Check sheet for the modelled part. Datum: model origin and axes. Units: mm. Round coordinates to 2 decimals unless told otherwise and drop trailing zeros. Write each loop counter-clockwise with the first axis right and the second up, starting at its lowest first coordinate (ties: lowest second). Pieces come first, ordered by that corner, then holes. Notation, with made-up numbers: M 68,43.25 L 75,43.25 A31 cw 75,76.25 Z; hole C 2,6.25 d3. An arc over 180 degrees is marked long. Answer in a Markdown table with one row per item.
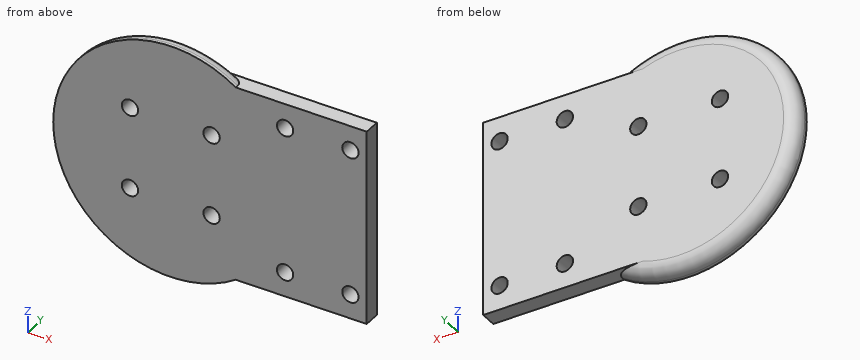
```python
from build123d import *

# Parameters (mm, degrees)
EXTRUDE_1_DEPTH     = 5
FILLET_1_R          = 4
SKETCH_2_R          = 2.5
CUT_EXTRUDE_1_DEPTH = 71.149839773


with BuildPart() as part:
    # 草图1 → 凸台-拉伸1 (new body)
    with BuildSketch(Plane(origin=(0, 0, 0), x_dir=(1, 0, 0), z_dir=(0, 1, 0))):
        with BuildLine():
            Line((19.899748742, -30), (60, -30))
            Line((60, -30), (60, 30))
            Line((60, 30), (19.899748742, 30))
            ThreePointArc((19.899748742, 30), (-36, 0), (19.899748742, -30))
        make_face()
    extrude(amount=EXTRUDE_1_DEPTH)

    # 圆角1
    fillet_1_edges = [part.edges().sort_by_distance(p)[0] for p in [
        (-36, 5, 0),
    ]]
    fillet(fillet_1_edges, radius=FILLET_1_R)

    # 草图2 → 切除-拉伸1 (cut, through all)
    with BuildSketch(Plane(origin=(0, 5, 0), x_dir=(1, 0, 0), z_dir=(0, 1, 0))):
        with Locations(Location((-12.5, 12.5, 0), (0, 0, 270))):
            Circle(SKETCH_2_R)
        with Locations(Location((12.5, 12.5, 0), (0, 0, 270))):
            Circle(SKETCH_2_R)
        with Locations(Location((12.5, -12.5, 0), (0, 0, 270))):
            Circle(SKETCH_2_R)
        with Locations(Location((-12.5, -12.5, 0), (0, 0, 270))):
            Circle(SKETCH_2_R)
        with Locations(Location((35, 22.5, 0), (0, 0, 270))):
            Circle(SKETCH_2_R)
        with Locations(Location((55, 22.5, 0), (0, 0, 270))):
            Circle(SKETCH_2_R)
        with Locations(Location((55, -22.5, 0), (0, 0, 270))):
            Circle(SKETCH_2_R)
        with Locations(Location((35, -22.5, 0), (0, 0, 270))):
            Circle(SKETCH_2_R)
    extrude(amount=-CUT_EXTRUDE_1_DEPTH, mode=Mode.SUBTRACT)


solid = part.part
```
1. Section check D-D, the plane x = 39.5. Record the cut outline in (y, z).
Found:
| item | result |
|---|---|
| outline | M 0,-30 L 5,-30 L 5,30 L 0,30 Z |
2. Scan lines: L1, parallel to X at y = 2.1, z = -22.5; L2, parallel to X at y = 3, z = -12.5; L3, parallel to Z at x = 11, y = 1.8. Record each from-to range of solid material in increasing order.
Found:
| item | result |
|---|---|
| L1 | x = -27.9 to 32.5, 37.5 to 52.5, 57.5 to 60 |
| L2 | x = -33.19 to -15, -10 to 10, 15 to 60 |
| L3 | z = -34.19 to -14.5, -10.5 to 10.5, 14.5 to 34.19 |
3. Go/stop test with flat-tipped pins: pin 1 (3 mm diameter, centred on x = 55, z = -22.5, fed in from -Y); pin 2 (2 mm diameter, centred on y = 1.5, z = -16.5, fed in from -X); pin 3 (2 mm diameter, centred on x = 24.5, y = 1.5, fed in from -Z); pin 4 (3 mm diameter, centred on y = 4, z = -27.5, fed in from -X). Record where each tip stops, or that it passes through.
Found:
| item | result |
|---|---|
| pin 1 | passes through |
| pin 2 | stops at x = -32.47 |
| pin 3 | stops at z = -30 |
| pin 4 | stops at x = -23.7 |
4. Section check B-B, the plane y = 3.6. Count the separate pieces of the cut face and the enclosed holes in it, and give its area (3 significant figures).
Found:
| item | result |
|---|---|
| separate pieces | 1 |
| enclosed holes | 8 |
| area | 5,500 mm2 |
5. Section check A-A, the plane x = 55. Record the cut outline in (y, z).
Found:
| item | result |
|---|---|
| outline | M 0,-30 L 5,-30 L 5,-25 L 0,-25 Z; M 0,-20 L 5,-20 L 5,20 L 0,20 Z; M 0,25 L 5,25 L 5,30 L 0,30 Z |
